For this review, take the finished solid that the model builds, in its own axes (mm). A direction names the side the tool comes from. Round coordinates to 2 decimals unless told otherwise and drop trailing zeros. Loops run counter-clockwise (first coordinate to the right, second up) from the corner with the lowest first, then second, coordinate; pieces in that order, holes last. Notation, with made-up numbers: (-17.5, 85) -> (25.5, 85) arc R16 ccw to (25.5, 107) -> close; hole circle Ø10 at (-1.5, -12). An arc over 180 degrees is marked (long way). One line per question, with ' | ' between items. Start each with the question number.
1. Consider section C-C (x = -8.6). Count the separate pieces of the cut face and the enclosed holes in it, and give its area (3 significant figures).
2. For faces 1 (the face through (-8.244, 14.986, 43.056)), 2 (the face through (-11.531, -0.307, 42.965)), 3 (the face through (-10.01, 7.67, 22.2)), 4 (the face through (-14.45, -1.39, 43.11)), list the 3-axis set-ups (+Z, -Z, +X, -X, +Y, -Y) from which the entire face can be reached by the end or side of a thin tool; tool diameter is ignored.
3. For pin 1 Ø3 at (x, z) = (-2, 34) entering from -Y; pin 2 Ø1 at (y, z) = (17, 21) entering from -X; pin 3 Ø2.5 at (x, z) = (-1, 34.5) entering from +Y, all flat-tipped, find the tip position at first contact; note any pin that passes through.
4. Consider section B-B (y = 12.7). Write out the cut boundary in (x, z), and give its area (3 significant figures).
5. Wall thickness on line 1 along X through (y, z) = (2.5, 43.08); line 2 along Y through (x, z) = (0, 27.7); line 3 along X through (y, z) = (2.95, 43.08): over which ranges is each line inside the solid? List them lowest first.
6. Consider section A-A (z = 21). Write out the cut boundary in (x, y), and give its area (3 significant figures).
7. Draft analysis for pull direction X (two halves, no side actions). For faces 5 (the face through (8.396, -17.289, 35.056)), 6 (the face through (-2.799, -21.317, 34.014)), 7 (the face through (-10, 18, 43)), state which applies: pulls with the +X half, pulls with the -X half, needs draft (parallel to the pull), parting line crosses it, or undercut.
```python
from build123d import *

# Parameters (mm, degrees)
CUT_EXTRUDE_7_DEPTH        = 16
CUT_EXTRUDE_START          = -25.5
CUT_EXTRUDE_3_OUTLINE_R    = 9.5
CUT_EXTRUDE_3_DEPTH        = 25.5
CUT_EXTRUDE_4_DEPTH        = 8
SKETCH_18_R                = 1.25
CUT_EXTRUDE_10_DEPTH       = 5
HOLE_WIZARD_M31_AT_2_COUNT = 2
HOLE_WIZARD_M31_AT_2_PITCH = 26
CHAMFER_1_SIZE             = 4
SKETCH_20_R                = 1.8
CUT_EXTRUDE_1_DEPTH        = 43.725870383
CUT_EXTRUDE_12_DEPTH       = 15
CUT_EXTRUDE_13_DEPTH       = 13
CUT_EXTRUDE_START_2        = -11.2
CUT_EXTRUDE_14_DEPTH       = 16
CUT_EXTRUDE_15_DEPTH       = 59.390924036
CUT_EXTRUDE_15_DEPTH_BACK  = 59.390924036
SKETCH_30_W                = 26
SKETCH_30_H                = 1.6


# Read off the part's stored shape, not the designer's step: the extrude step
with BuildPart() as part:
    # Sketch 2 → Revolve 2 (revolve)
    with BuildSketch(Plane(origin=(0, 0, 0), x_dir=(0, 0, -1), z_dir=(1, 0, 0)), mode=Mode.PRIVATE) as revolve_2_sk:
        Polygon((-47, 9.5), (-22, 9.5), (-22, 21), (-14, 21), (-14, 20), (0, 20), (0, 24.5), (-33, 24.5), (-33, 21.5), (-35, 21.5), (-35, 24.5), (-47, 24.5), align=None)
    revolve(revolve_2_sk.sketch.rotate(Axis((0, 0, 0), (0, 0, -1)), 90), axis=Axis((0, 0, 0), (0, 0, -1)))

    # Sketch 11 → Cut-Extrude 7 (cut)
    with BuildSketch(Plane.XY.offset(47)):
        with BuildLine():
            Line((-4.2, -19), (4.2, -19))
            ThreePointArc((4.2, -19), (8.442640687, -17.242640687), (10.2, -13))
            Line((10.2, -13), (10.2, 3.1265006))
            ThreePointArc((10.2, 3.1265006), (9.360092406, 8.51845162), (4.5, 11))
            Line((4.5, 11), (-4.5, 11))
            ThreePointArc((-4.5, 11), (-9.360092406, 8.51845162), (-10.2, 3.1265006))
            Line((-10.2, 3.1265006), (-10.2, -13))
            ThreePointArc((-10.2, -13), (-8.442640687, -17.242640687), (-4.2, -19))
        make_face()
    extrude(amount=-CUT_EXTRUDE_7_DEPTH, mode=Mode.SUBTRACT)

    # Cut-Extrude 3 outline → Cut-Extrude 3 (cut)
    with BuildSketch(Plane(origin=(0, 0, 0), x_dir=(-1, 0, 0), z_dir=(0, 0, -1)).offset(CUT_EXTRUDE_START)):
        with BuildLine():
            ThreePointArc((6.060829661, -23.738499191), (17.324116139, -17.324116139), (23.738499191, -6.060829661))
            Line((23.738499191, -6.060829661), (-6.060829661, 23.738499191))
            ThreePointArc((-6.060829661, 23.738499191), (-17.324116139, 17.324116139), (-23.738499191, 6.060829661))
            Line((-23.738499191, 6.060829661), (6.060829661, -23.738499191))
        make_face()
        Circle(CUT_EXTRUDE_3_OUTLINE_R, mode=Mode.SUBTRACT)
    extrude(amount=CUT_EXTRUDE_3_DEPTH, mode=Mode.SUBTRACT)

    # Sketch 5 → Cut-Extrude 4 (cut)
    with BuildSketch(Plane.XY.offset(47)):
        with BuildLine():
            Line((17, 5), (17, 1.737387097))
            Line((17, 1.737387097), (12, -12))
            Line((12, -12), (10.2, -12))
            Line((10.2, -12), (10.2, -13))
            ThreePointArc((10.2, -13), (8.442640687, -17.242640687), (4.2, -19))
            Line((4.2, -19), (-4.2, -19))
            ThreePointArc((-4.2, -19), (-8.442640687, -17.242640687), (-10.2, -13))
            Line((-10.2, -13), (-10.2, -9.827820985))
            Line((-10.2, -9.827820985), (-16.587454885, -14.300365046))
            Line((-16.587454885, -14.300365046), (-24.273530206, -3.323511896))
            ThreePointArc((-24.273530206, -3.323511896), (1.66560949, -24.443316981), (24.5, 0))
            ThreePointArc((24.5, 0), (2.513258562, 24.370751556), (-23.98436991, 5))
            Line((-23.98436991, 5), (-10.5, 5))
            ThreePointArc((-10.5, 5), (-8.742640687, 9.242640687), (-4.5, 11))
            Line((-4.5, 11), (4.5, 11))
            ThreePointArc((4.5, 11), (8.742640687, 9.242640687), (10.5, 5))
            Line((10.5, 5), (17, 5))
        make_face()
        Polygon((-10, 20), (7, 20), (7, 14), (-6.535898385, 14), (-10, 16), align=None, mode=Mode.SUBTRACT)
    extrude(amount=-CUT_EXTRUDE_4_DEPTH, mode=Mode.SUBTRACT)

    # Sketch 18 → Cut-Extrude 10 (cut)
    with BuildSketch(Plane(origin=(0, 5, 0), x_dir=(1, 0, 0), z_dir=(0, 1, 0))):
        with Locations(Location((-13.2, -43.08, 0), (0, 0, 180))):
            Circle(SKETCH_18_R)
        with Locations(Location((12.8, -43.08, 0), (0, 0, 180))):
            Circle(SKETCH_18_R)
    extrude(amount=-CUT_EXTRUDE_10_DEPTH, mode=Mode.SUBTRACT)

    # Sketch 24 → Hole Wizard M31 (revolve, cut)
    with BuildSketch(Plane(origin=(-13.2, 5, 43.08), x_dir=(0, 0, 1), z_dir=(1, 0, 0))):
        Polygon((0, 0), (0, 9.251075774), (1.25, 8.5), (1.25, 6), (1.5, 6), (1.5, 0.25), (1.75, 0), align=None)
    hole_wizard_m31 = revolve(axis=Axis((-13.2, 11.35, 43.08), (0, -1, 0)), mode=Mode.SUBTRACT)

    # Hole Wizard M31 at 2: Hole Wizard M31 ×2
    with Locations(*[(i * HOLE_WIZARD_M31_AT_2_PITCH, 0, 0) for i in range(1, HOLE_WIZARD_M31_AT_2_COUNT)]):
        add(hole_wizard_m31, mode=Mode.SUBTRACT)

    # Chamfer 1
    chamfer_1_edges = [part.edges().sort_by_distance(p)[0] for p in [
        (17, 3.368693549, 47),
    ]]
    chamfer(chamfer_1_edges, length=CHAMFER_1_SIZE)

    # Sketch 20 → Cut-Extrude 1 (cut, through all)
    with BuildSketch(Plane(origin=(0, 0, 22), x_dir=(-1, 0, 0), z_dir=(0, 0, -1))):
        with Locations((8.6, 12.7)):
            Circle(SKETCH_20_R)
    extrude(amount=-CUT_EXTRUDE_1_DEPTH, mode=Mode.SUBTRACT)

    # Sketch 21 → Hole Wizard M21 (revolve, cut)
    with BuildSketch(Plane(origin=(2, 20, 43), x_dir=(0, 0, 1), z_dir=(1, 0, 0))):
        Polygon((0, 0), (0, 6), (1.1, 6), (0.8, 5.826794919), (0.8, 0.173205081), (1.1, 0), align=None)
    revolve(axis=Axis((2, 26.35, 43), (0, -1, 0)), mode=Mode.SUBTRACT)

    # Sketch 23 → Cut-Extrude 12 (cut)
    with BuildSketch(Plane(origin=(4.75, -8.227241336, 0), x_dir=(0, 0, -1), z_dir=(-0.499999999999998, 0.8660254037844398, 0))):
        with BuildLine():
            Line((-40.5, 11.5), (-40.5, 4.634817269))
            Line((-40.5, 4.634817269), (-45.5, 4.634817269))
            Line((-45.5, 4.634817269), (-45.5, 11.5))
            ThreePointArc((-45.5, 11.5), (-43, 14), (-40.5, 11.5))
        make_face()
    extrude(amount=CUT_EXTRUDE_12_DEPTH, mode=Mode.SUBTRACT)

    # Sketch 26 → Cut-Extrude 13 (cut)
    with BuildSketch(Plane(origin=(-3.249191362, -8.927079897, 0), x_dir=(0, 0, 1), z_dir=(0.3420201433256694, 0.9396926207859083, 0))):
        with BuildLine():
            Line((45.5, 10.5), (45.5, 4.710471755))
            Line((45.5, 4.710471755), (40.5, 4.710471755))
            Line((40.5, 4.710471755), (40.5, 10.5))
            ThreePointArc((40.5, 10.5), (43, 13), (45.5, 10.5))
        make_face()
    extrude(amount=CUT_EXTRUDE_13_DEPTH, mode=Mode.SUBTRACT)

    # Sketch 27 → Cut-Extrude 14 (cut)
    with BuildSketch(Plane(origin=(1.26186816, -1.802134497, 0), x_dir=(0.8191520442889928, 0.5735764363510447, 0), z_dir=(0.5735764363510447, -0.8191520442889928, 0)).offset(CUT_EXTRUDE_START_2)):
        with BuildLine():
            Line((-18.79, 40), (-27.979598057, 40))
            Line((-27.979598057, 40), (-27.979598057, 48.487247608))
            Line((-27.979598057, 48.487247608), (-15.79, 48.487247608))
            Line((-15.79, 48.487247608), (-15.79, 43))
            ThreePointArc((-15.79, 43), (-16.668679656, 40.878679656), (-18.79, 40))
        make_face()
    extrude(amount=-CUT_EXTRUDE_14_DEPTH, mode=Mode.SUBTRACT)

    # Sketch 28 → Hole Wizard 2-561 (revolve, cut)
    with BuildSketch(Plane(origin=(-20.963630861, -3.691921059, 43), x_dir=(-0.8191520442889927, -0.5735764363510447, 0), z_dir=(0, 0, 1))):
        Polygon((0, 0), (0, 11.2), (1.397, 11.2), (0.889, 10.844294571), (0.889, 0.355705429), (1.397, 0), align=None)
    revolve(axis=Axis((-24.605841232, 1.509694423, 43), (0.5735764363510447, -0.8191520442889927, 0)), mode=Mode.SUBTRACT)

    # Sketch 30 → Cut-Extrude 15 (cut, two sides: drawn at the far end of the back side and taken through both)
    with BuildSketch(Plane(origin=(0, 0, 0), x_dir=(-0.7071067811865464, 0.7071067811865488, 0), z_dir=(0.7071067811865488, 0.7071067811865464, 0)).offset(-CUT_EXTRUDE_15_DEPTH_BACK)):
        with Locations((0, 25.2)):
            Rectangle(SKETCH_30_W, SKETCH_30_H)
    extrude(amount=CUT_EXTRUDE_15_DEPTH + CUT_EXTRUDE_15_DEPTH_BACK, mode=Mode.SUBTRACT)


solid = part.part
```
Answer block:
1) separate pieces: 3 | enclosed holes: 0 | area: 462 mm2
2) face 1: +Z, -X, -Y | face 2: none | face 3: -Z | face 4: +Y
3) pin 1: stops at y = -24.48 | pin 2: stops at x = -18.11 | pin 3: stops at y = 24.5
4) outline: (-20.95, 0) -> (-15.45, 0) -> (-15.45, 14) -> (-16.72, 14) -> (-16.72, 22) -> (-10.4, 22) -> (-10.4, 39) -> (-20.95, 39) -> (-20.95, 35) -> (-17.35, 35) -> (-17.35, 33) -> (-20.95, 33) -> close; (-6.8, 22) -> (-4.98, 22) -> (-4.98, 24.4) -> (-5.68, 24.4) -> (-5.68, 26) -> (20.95, 26) -> (20.95, 33) -> (17.35, 33) -> (17.35, 35) -> (20.95, 35) -> (20.95, 39) -> (-6.8, 39) -> close | area: 643 mm2
5) line 1: x = -21.03 to -14.7, -11.7 to -10.2, 10.2 to 11.3, 14.3 to 16.92 | line 2: y = -24.5 to -9.5, 9.5 to 24.5 | line 3: x = -21.34 to -14.7, -11.7 to -10.2, 10.2 to 11.3, 14.3 to 16.92
6) outline: (-23.74, -6.06) -> (-20.77, -3.09) arc R21 cw to (3.09, 20.77) -> (6.06, 23.74) arc R24.5 ccw to start; (-6.06, -23.74) arc R24.5 ccw to (23.74, 6.06) -> (20.77, 3.09) arc R21 cw to (-3.09, -20.77) -> close | area: 315 mm2
7) face 5: undercut | face 6: parting line crosses it | face 7: pulls with the -X half
